Source: CAD feature listing. Evaluate the final solid. Frame: model axes, mm. Face numbers are marked on the shaded views. A direction names the side the tool comes from. Round coordinates to 2 decimals unless told otherwise and drop trailing zeros. Loops run counter-clockwise (first coordinate to the right, second up) from the corner with the lowest first, then second, coordinate; pieces in that order, holes last. Notation, with made-up numbers: (70.25, 7) - (115.25, 7) arc R28 cw to (115.25, 43) - close; hole circle Ø8 at (-18.75, -23.75). An arc over 180 degrees is marked (long way). Write item = value, one per line. Start each with the question number.
from build123d import *

# Parameters (mm, degrees)
SKETCH2_R           = 2.25
BOSS_EXTRUDE1_DEPTH = 75
SKETCH3_R           = 3
BOSS_EXTRUDE2_DEPTH = 1
BOSS_EXTRUDE3_START = 5
SKETCH4_R           = 2.25
BOSS_EXTRUDE3_DEPTH = 5


with BuildPart() as part:
    # Sketch2 → Boss-Extrude1 (new body)
    with BuildSketch(Plane.XY):
        Circle(SKETCH2_R)
    extrude(amount=BOSS_EXTRUDE1_DEPTH)

    # Sketch3 → Boss-Extrude2 (add)
    with BuildSketch(Plane(origin=(0, 0, 0), x_dir=(-1, 0, 0), z_dir=(0, 0, -1))):
        Circle(SKETCH3_R)
    extrude(amount=BOSS_EXTRUDE2_DEPTH)

    # Sketch4 → Boss-Extrude3 (add)
    with BuildSketch(Plane(origin=(0, 0, -1), x_dir=(-1, 0, 0), z_dir=(0, 0, -1)).offset(BOSS_EXTRUDE3_START)):
        with Locations(Location((0, 0, 0), (0, 0, 180))):
            Circle(SKETCH4_R)
    extrude(amount=-BOSS_EXTRUDE3_DEPTH)


solid = part.part
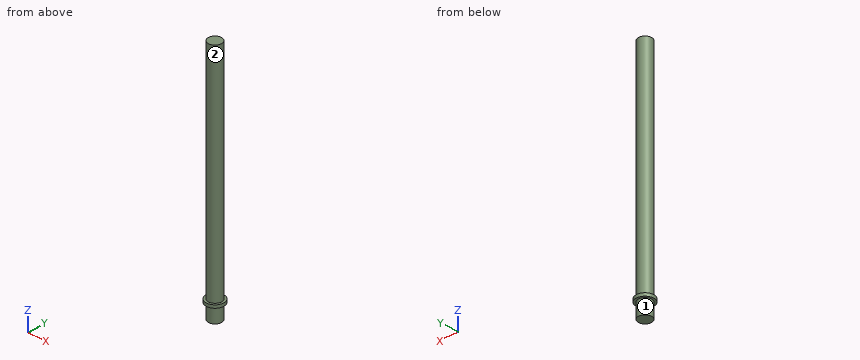
(1) Pin query (flat end, axial travel): P1, Ø1.5, axis at y = 1.5, z = 63.5, coming from the -X side. Return the tip coordinate at first contact, or that it passes through.
(2) Cut plane C-C (z = 10). Output: boundary loops of the cut face in (x, y).
(3) Cut plane A-A (x = 0). Output: boundary loops of the cut face in (y, z).
(4) Material intervals for line 1 along Y through (x, z) = (0, 21.5); line 2 along Z through (x, y) = (-2.7, -0.3); line 3 along X through (y, z) = (-2, 55), sorted ascending. Write a range as from..to.
(5) Access query for the marked faces 1 and 2. Directions: +Z, -Z, +X, -X, +Y, -Y. A direction counts if a zero-diameter tool reaches every point of the face in a straight line with its end or side. Return the directions, or none.
Solution:
q1.P1 = -2.12
q2.outline = circle Ø4.5 at (0, 0)
q3.outline = (-3, -1) - (-2.25, -1) - (-2.25, -6) - (2.25, -6) - (2.25, -1) - (3, -1) - (3, 0) - (2.25, 0) - (2.25, 75) - (-2.25, 75) - (-2.25, 0) - (-3, 0) - close
q4.line_1 = -2.25..2.25
q4.line_2 = -1..0
q4.line_3 = -1.03..1.03
q5.face_1 = -Z
q5.face_2 = +Z
